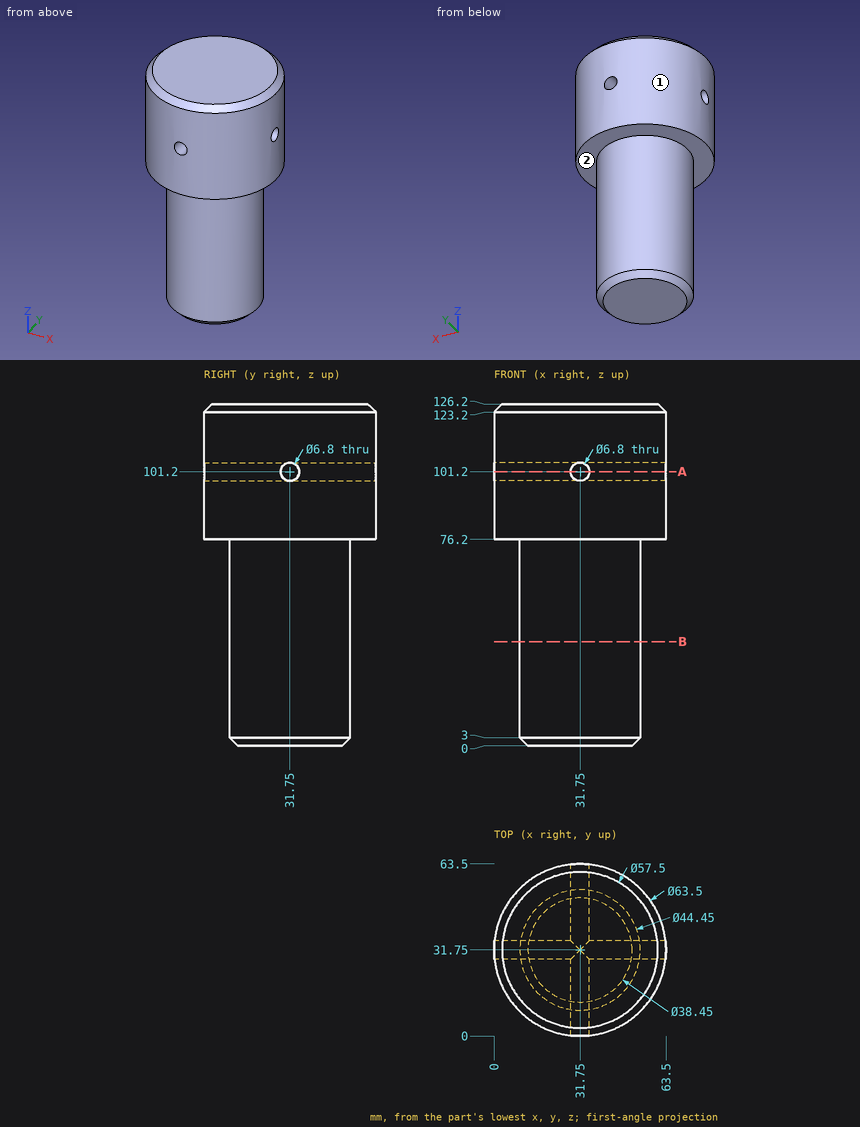
The figure shows three views and two pictorial views of one solid part (mm, origin at its lowest corner). Answer the questions. A direction names the side the tool comes from. Give positions to 0.01 mm unless a question says otherwise; leave off trailing zeros. Loops run counter-clockwise (first coordinate to the right, second up) from the corner with the lowest first, then second, coordinate; pieces in that order, holes last. Notation, with made-up numbers: (30, 23) -> (62, 23) arc R9 ccw to (62, 27) -> close; hole circle Ø1 at (28, 37.5). An arc over 180 degrees is marked (long way). Put each result on its own line as item: value. Start each with the question number.
Item 1: Find the intervals of material crossed by L1, parallel to Z at x = 4.5, y = 31.5; L2, parallel to Z at x = 31.75, y = 23; L3, parallel to Z at x = 41.5, y = 6, in increasing order. Write a range as [from, to].
Item 2: Which of the six approach directions +Z, -Z, +X, -X, +Y, -Y give full straight-line access (tool end or side, diameter ignored) to the marked faces 1 and 2?
Item 3: The part is cut by section B-B (z = 38.5). Give the vertices of the cut face in (x, y) (3 decimals).
Item 4: Each of these flat-tipped pins is pushed along its axis until it touches: P1, Ø3, axis at y = 18, z = 88, coming from the +X side; P2, Ø2, axis at x = 41.5, y = 51, coming from the -Z side; P3, Ø4, axis at y = 13.5, z = 22.5, coming from the +X side; P4, Ø1.5, axis at y = 33, z = 103, coming from the +X side (3 decimals). Where does it stop, or does it pass through?
Item 5: The part is cut by section A-A (z = 101.2). Give the vertices of the cut face in (x, y), then the cut area to 3 significant figures.
Answers below:
1. L1: [76.2, 97.81], [104.59, 126.2]
1. L2: [0, 97.8], [104.6, 126.2]
1. L3: [76.2, 126.2]
2. face 1: +Z, -Z
2. face 2: -Z
3. outline: circle Ø44.45 at (31.75, 31.75)
4. P1: x = 61.04
4. P2: z = 1.35
4. P3: x = 46.91
4. P4: through
5. outline: (0.18, 28.35) arc R31.75 ccw to (28.35, 0.18) -> (28.35, 28.35) -> close; (0.18, 35.15) -> (28.35, 35.15) -> (28.35, 63.32) arc R31.75 ccw to start; (35.15, 0.18) arc R31.75 ccw to (63.32, 28.35) -> (35.15, 28.35) -> close; (35.15, 35.15) -> (63.32, 35.15) arc R31.75 ccw to (35.15, 63.32) -> close
5. area: 2,350 mm2
